```python
from build123d import *
from build123d.topology import SkipClean

# Parameters (mm, degrees)
ESTRUSIONE_ESTRUSIONE1_DEPTH = 40
RACCORDO1_R                  = 7
SCHIZZO2_W                   = 4
SCHIZZO2_H                   = 20
TAGLIO_ESTRUSIONE1_DEPTH     = 40
SCHIZZO3_R                   = 1.05
SCHIZZO3_R_2                 = 3.5
TAGLIO_ESTRUSIONE2_DEPTH     = 40
SCHIZZO4_R                   = 2.5
SCHIZZO4_R_2                 = 1.05
ESTRUSIONE_ESTRUSIONE2_DEPTH = 3
RACCORDO2_R                  = 2
SCHIZZO5_R                   = 1.5
TAGLIO_ESTRUSIONE3_DEPTH     = 17
TAGLIO_ESTRUSIONE4_DEPTH     = 10
RACCORDO3_R                  = 5
RACCORDO4_R                  = 5


with BuildPart() as part:
    # Schizzo1 → Estrusione-Estrusione1 (new body)
    with BuildSketch(Plane.XY):
        Polygon((0, 0), (-40, 0), (-29.647238196, 38.637033052), (-33.510941501, 39.672309232), (-45.212901491, -4), (0, -4), align=None)
    extrude(amount=ESTRUSIONE_ESTRUSIONE1_DEPTH)

    # Raccordo1
    raccordo1_edges = [part.edges().sort_by_distance(p)[0] for p in [
        (-45.212901491, -4, 20),
        (-40, 0, 20),
    ]]
    fillet(raccordo1_edges, radius=RACCORDO1_R)

    # Schizzo2 → Taglio-Estrusione1 (cut)
    with BuildSketch(Plane(origin=(0, 0, 0), x_dir=(1, 0, 0), z_dir=(0, 1, 0))):
        with Locations((-28.87742239, -20)):
            Rectangle(SCHIZZO2_W, SCHIZZO2_H)
    extrude(amount=-TAGLIO_ESTRUSIONE1_DEPTH, mode=Mode.SUBTRACT)

    # Schizzo3 → Taglio-Estrusione2 (cut)
    with BuildSketch(Plane(origin=(-41.184211381, 11.03527618, 0), x_dir=(0, 0, 1), z_dir=(-0.9659258262890673, 0.2588190451025247, 0))):
        with Locations(Location((30.402866557, 25.309568218, 0), (0, 0, 270))):
            Circle(SCHIZZO3_R)
        with Locations(Location((9.20859967, 25.309568218, 0), (0, 0, 270))):
            Circle(SCHIZZO3_R)
        with Locations(Location((30.402866557, 13.009568218, 0), (0, 0, 270))):
            Circle(SCHIZZO3_R)
        with Locations(Location((9.20859967, 13.009568218, 0), (0, 0, 270))):
            Circle(SCHIZZO3_R)
        with Locations(Location((19.902866557, 13.409568216, 0), (0, 0, 270))):
            Circle(SCHIZZO3_R_2)
    extrude(amount=-TAGLIO_ESTRUSIONE2_DEPTH, mode=Mode.SUBTRACT)

    # Schizzo4 → Estrusione-Estrusione2 (add)
    # profile 1 of 4: a face of its own
    with SkipClean():  # the faces are left unmerged after this step: merging them gives an invalid solid
        with BuildSketch(Plane(origin=(-37.320508076, 10, 0), x_dir=(0, 0, -1), z_dir=(0.9659258262890674, -0.2588190451025245, 0))):
            with Locations(Location((-9.20859967, 13.009568218, 0), (0, 0, 270))):
                Circle(SCHIZZO4_R)
            with Locations(Location((-9.20859967, 13.009568218, 0), (0, 0, 90))):
                Circle(SCHIZZO4_R_2, mode=Mode.SUBTRACT)
        # profile 2 of 4: a face of its own
        with BuildSketch(Plane(origin=(-37.320508076, 10, 0), x_dir=(0, 0, -1), z_dir=(0.9659258262890674, -0.2588190451025245, 0))):
            with Locations(Location((-30.402866557, 13.009568218, 0), (0, 0, 270))):
                Circle(SCHIZZO4_R)
            with Locations(Location((-30.402866557, 13.009568218, 0), (0, 0, 270))):
                Circle(SCHIZZO4_R_2, mode=Mode.SUBTRACT)
        # profile 3 of 4: a face of its own
        with BuildSketch(Plane(origin=(-37.320508076, 10, 0), x_dir=(0, 0, -1), z_dir=(0.9659258262890674, -0.2588190451025245, 0))):
            with Locations(Location((-30.402866557, 25.309568218, 0), (0, 0, 270))):
                Circle(SCHIZZO4_R)
            with Locations(Location((-30.402866557, 25.309568218, 0), (0, 0, 270))):
                Circle(SCHIZZO4_R_2, mode=Mode.SUBTRACT)
        # profile 4 of 4: a face of its own
        with BuildSketch(Plane(origin=(-37.320508076, 10, 0), x_dir=(0, 0, -1), z_dir=(0.9659258262890674, -0.2588190451025245, 0))):
            with Locations(Location((-9.20859967, 25.309568218, 0), (0, 0, 270))):
                Circle(SCHIZZO4_R)
            with Locations(Location((-9.20859967, 25.309568218, 0), (0, 0, 90))):
                Circle(SCHIZZO4_R_2, mode=Mode.SUBTRACT)
        extrude(amount=ESTRUSIONE_ESTRUSIONE2_DEPTH)
    add(part.part.scale(1), mode=Mode.REPLACE)  # the faces are merged on a copy

    # Raccordo2
    raccordo2_edges = [part.edges().sort_by_distance(p)[0] for p in [
        (-33.306336439, 24.981092497, 9.20859967),
        (-33.306336439, 24.981092497, 30.402866557),
        (-30.122862185, 36.86198016, 30.402866557),
        (-30.122862185, 36.86198016, 9.20859967),
    ]]
    fillet(raccordo2_edges, radius=RACCORDO2_R)

    # Schizzo5 → Taglio-Estrusione3 (cut)
    with BuildSketch(Plane(origin=(0, 0, 0), x_dir=(1, 0, 0), z_dir=(0, 1, 0))):
        with Locations(Location((-2.444220089, -36.8336475, 0), (0, 0, 180))):
            Circle(SCHIZZO5_R)
        with Locations(Location((-2.444220089, -3.1663525, 0), (0, 0, 180))):
            Circle(SCHIZZO5_R)
        with Locations(Location((-28.433202301, -3.1663525, 0), (0, 0, 180))):
            Circle(SCHIZZO5_R)
        with Locations(Location((-28.433202301, -36.8336475, 0), (0, 0, 180))):
            Circle(SCHIZZO5_R)
    extrude(amount=-TAGLIO_ESTRUSIONE3_DEPTH, mode=Mode.SUBTRACT)

    # Schizzo6 → Taglio-Estrusione4 (cut)
    with BuildSketch(Plane(origin=(0, 0, 0), x_dir=(1, 0, 0), z_dir=(0, 1, 0))):
        Polygon((0, -20), (0, -30), (-3, -30), (-3, -10), (0, -10), align=None)
    extrude(amount=-TAGLIO_ESTRUSIONE4_DEPTH, mode=Mode.SUBTRACT)

    # Raccordo3
    # the kernel refuses this fillet: 5 mm, written as the material it takes off along each edge
    with BuildSketch(Plane(origin=(0, 11.456439237, 10), x_dir=(0, 0, -1), z_dir=(0, -1, 0))) as raccordo3_piece_1:
        with BuildLine():
            CenterArc((4.582575695, -5), RACCORDO3_R, 90, 66.421821522)
            Line((0, -3), (-0.091651514, -2.96))
            ThreePointArc((-0.091651514, -2.96), (-0.1, -1.5), (-0.1, 0))
            Line((-0.1, 0), (0, 0.1))
            Line((0, 0.1), (4.582575695, 0.1))
            Line((4.582575695, 0.1), (4.582575695, 0))
        make_face()
    extrude(amount=26.912878475, mode=Mode.SUBTRACT)
    with BuildSketch(Plane(origin=(0, 11.456439237, 30), x_dir=(0, 0, 1), z_dir=(0, -1, 0))) as raccordo3_piece_2:
        with BuildLine():
            CenterArc((4.582575695, 5), RACCORDO3_R, 203.578178478, 66.421821522)
            Line((0, 3), (-0.091651514, 2.96))
            ThreePointArc((-0.091651514, 2.96), (-0.1, 1.5), (-0.1, 0))
            Line((-0.1, 0), (0, -0.1))
            Line((0, -0.1), (4.582575695, -0.1))
            Line((4.582575695, -0.1), (4.582575695, 0))
        make_face()
    extrude(amount=26.912878475, mode=Mode.SUBTRACT)

    # Raccordo4
    raccordo4_edges = [part.edges().sort_by_distance(p)[0] for p in [
        (-3, -2, 30),
        (-3, -2, 10),
    ]]
    fillet(raccordo4_edges, radius=RACCORDO4_R)


solid = part.part
```
Part model, mm, in its own coordinate system. A direction names the side the tool comes from. Round coordinates to 2 decimals unless told otherwise and drop trailing zeros. Loops run counter-clockwise (first coordinate to the right, second up) from the corner with the lowest first, then second, coordinate; pieces in that order, holes last. Notation, with made-up numbers: (-6.5, 18.25) -> (2.5, 18.25) arc R15 cw to (2.5, 29.25) -> close; hole circle Ø5 at (61, 78). An arc over 180 degrees is marked (long way). Use a Markdown table: item, result.
1) Cut at D-D, the plane y = 11. List the corners of the cut face in (x, z).
The answers:
| item | result |
|---|---|
| outline | (-41.19, 0) -> (-37.05, 0) -> (-37.05, 40) -> (-41.19, 40) -> close |
2) Tool access for faces 1 (the flat face through (-26.877, -2, 20)), 2 (the flat face through (-33.699, 23.516, 15.276)), 3 (the flat face through (-28, 33.2, 31.5)), 4 (the flat face through (-3, -2, 20)), 5 (the cylindrical face through (-26.935, -1.972, 3.232)): list every direction of +Z, -Z, +X, -X, +Y, -Y with a clear straight run to the whole face (end or side of a thin tool).
The answers:
| item | result |
|---|---|
| face 1 | +Y, -Y |
| face 2 | +X |
| face 3 | +Z, -Z, +X |
| face 4 | +X, +Y, -Y |
| face 5 | -Y |
3) Cut at A-A, the plane z = 15. List the corners of the cut face in (x, y), and give its area (3 significant figures).
The answers:
| item | result |
|---|---|
| outline | (-42.85, 4.81) arc R7 ccw to (-36.09, -4) -> (-30.88, -4) -> (-30.88, 0) arc R7 cw to (-37.64, 8.81) -> (-29.65, 38.64) -> (-33.51, 39.67) -> close; (-26.88, -4) -> (-3, -4) -> (-3, 0) -> (-26.88, 0) -> close |
| area | 313 mm2 |
4) Pull direction Z, two halves, no side cores. Call faces 6 (the cylindrical face through (-31.89, 20.62, 7.1)), 7 (the flat face through (-38, 11, 40)), 8 (the cylindrical face through (-1.34, -1.97, 37.85)), 9 (the flat face through (-18, -4, 20)): pulls with the +Z half, pulls with the -Z half, needs draft (parallel to the pull), parting line crosses it, or undercut.
The answers:
| item | result |
|---|---|
| face 6 | undercut |
| face 7 | pulls with the +Z half |
| face 8 | undercut |
| face 9 | needs draft |
5) Drop flat-ended pins along their axis: pin 1 Ø1.8 at (x, z) = (-28.43, 3.17) entering from -Y; pin 2 Ø2 at (y, z) = (-1.5, 23.5) entering from +X; pin 3 Ø3.5 at (x, z) = (-2.44, 3.17) entering from +Y; pin 4 Ø5 at (y, z) = (2, 10) entering from +X. Give the stop position or say it passes through.
The answers:
| item | result |
|---|---|
| pin 1 | passes through |
| pin 2 | stops at x = -3 |
| pin 3 | stops at y = 0 |
| pin 4 | stops at x = -1.06 |
6) Probe line 1 (Y direction, x = -25, z = 17); line 2 (X direction, y = 32.5, z = 21); line 3 (X direction, y = 20.5, z = 7). List the from-to ranges inside material, lowest first. Write a range as [from, to].
The answers:
| item | result |
|---|---|
| line 1 | y = [-4, 0] |
| line 2 | x = [-35.43, -31.29] |
| line 3 | x = [-38.65, -33.73] |
7) Cut at C-C, the plane x = -6. List the corners of the cut face in (y, z), and give its area (3 significant figures).
The answers:
| item | result |
|---|---|
| outline | (-4, 0) -> (0, 0) -> (0, 40) -> (-4, 40) -> close |
| area | 160 mm2 |
8) Cut at B-B, the plane y = -1. List the corners of the cut face in (x, z).
The answers:
| item | result |
|---|---|
| outline | (-41.83, 0) -> (0, 0) -> (0, 5.42) arc R5 ccw to (-1.5, 8.99) arc R5 cw to (-3, 12.56) -> (-3, 27.44) arc R5 cw to (-1.5, 31.01) arc R5 ccw to (0, 34.58) -> (0, 40) -> (-41.83, 40) -> close; hole (-30.88, 10) -> (-26.88, 10) -> (-26.88, 30) -> (-30.88, 30) -> close; hole circle Ø3 at (-28.43, 3.17); hole circle Ø3 at (-28.43, 36.83); hole circle Ø3 at (-2.44, 3.17); hole circle Ø3 at (-2.44, 36.83) |
